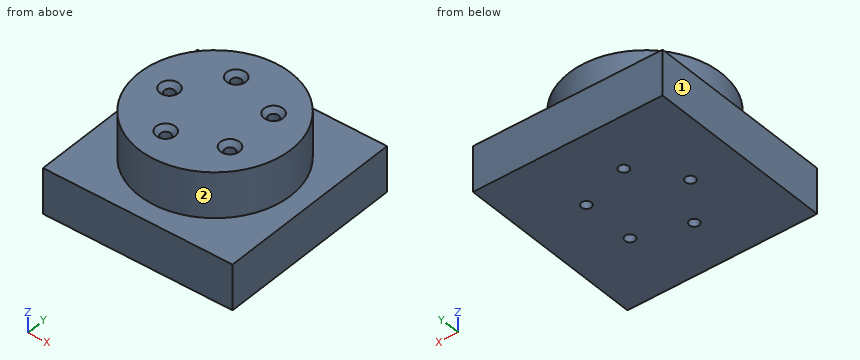
```python
from build123d import *

# Parameters (mm, degrees)
SKETCH1_W                                       = 125
SKETCH1_H                                       = 125
BOSS_EXTRUDE1_DEPTH                             = 30
SKETCH1_3_R                                     = 50
BOSS_EXTRUDE2_DEPTH                             = 30
CSK_FOR_M6_FLAT_HEAD_MACHINE_SCREW1_D           = 6.6
CSK_FOR_M6_FLAT_HEAD_MACHINE_SCREW1_CSINK_D     = 12.6
CSK_FOR_M6_FLAT_HEAD_MACHINE_SCREW1_CSINK_ANGLE = 90
CIRPATTERN1_COUNT                               = 5


with BuildPart() as part:
    # Sketch1 → Boss-Extrude1 (new body)
    with BuildSketch(Plane.XY):
        Rectangle(SKETCH1_W, SKETCH1_H)
    extrude(amount=-BOSS_EXTRUDE1_DEPTH)

    # Sketch1_3 → Boss-Extrude2 (add)
    with BuildSketch(Plane.XY):
        Circle(SKETCH1_3_R)
    extrude(amount=BOSS_EXTRUDE2_DEPTH)

    # CSK for M6 Flat Head Machine Screw1 (through all)
    with Locations(Plane.XY.offset(30)):
        with Locations((-30, 0)):
            csk_for_m6_flat_head_machine_screw1 = CounterSinkHole(CSK_FOR_M6_FLAT_HEAD_MACHINE_SCREW1_D / 2, CSK_FOR_M6_FLAT_HEAD_MACHINE_SCREW1_CSINK_D / 2, counter_sink_angle=CSK_FOR_M6_FLAT_HEAD_MACHINE_SCREW1_CSINK_ANGLE)

    # CirPattern1: CSK for M6 Flat Head Machine Screw1 ×5 about axis
    cirpattern1_axis = Axis((0, 0, 0), (0, 0, 1))
    for i in range(1, CIRPATTERN1_COUNT):
        add(csk_for_m6_flat_head_machine_screw1.rotate(cirpattern1_axis, i * 360 / CIRPATTERN1_COUNT), mode=Mode.SUBTRACT)


solid = part.part
```
The model under review builds one solid part; all positions refer to its coordinate system, in mm. Face numbers are marked on the shaded views. A direction names the side the tool comes from. Give positions to 0.01 mm unless a question says otherwise; leave off trailing zeros. Order: outer loops, then holes, each group sorted by start corner. A loop starts at its lowest first (then second) coordinate and runs counter-clockwise, first axis right, second up. Notation, with made-up numbers: (32.25, -20.75) - (39.25, -20.75) arc R29 ccw to (39.25, 7.25) - close; hole circle Ø8 at (55, 86). An arc over 180 degrees is marked (long way). Use CSV: the item, a comma, the result in double quotes. Start each with the question number.
Q1. We need section A-A, the plane x = -30. Write out the cut boundary in (y, z).
Q2. To check wall thickness, follow line 1 along Y through (x, z) = (-30, -5.5); line 2 along X through (y, z) = (17.5, -25); line 3 along Y through (x, z) = (-8, -16.5). State the ranges of each line that lie inside material, in increasing order. Write a range as [from, to].
Q3. We need section B-B, the plane y = 0. Write out the cut boundary in (x, z), and give its area (4 significant figures).
Q4. We need section D-D, the plane z = 23.5. Write out the cut boundary in (x, y).
Q5. We need section C-C, the plane x = 0. Write out the cut boundary in (y, z).
Q6. Tool access review of the marked faces 1 and 2: name each direction out of +Z, -Z, +X, -X, +Y, -Y from which nothing blocks a thin tool from reaching the whole face with its end or side.
Q7. Clearance check with flat-ended pins moving along their axes: pin 1 Ø3 at (y, z) = (-9.5, 15.5) entering from -X; pin 2 Ø10.5 at (x, y) = (-9.27, 28.53) entering from +Z; pin 3 Ø5 at (x, z) = (44, 20) entering from -Y. State where each tip first meets the part, or that it passes through.
Outcome:
1,outline,"(-62.5, -30) - (-3.3, -30) - (-3.3, 27) - (-6.3, 30) - (-40, 30) - (-40, 0) - (-62.5, 0) - close; (3.3, -30) - (62.5, -30) - (62.5, 0) - (40, 0) - (40, 30) - (6.3, 30) - (3.3, 27) - close"
2,line 1,"y = [-62.5, -3.3], [3.3, 62.5]"
2,line 2,"x = [-62.5, 20.97], [27.57, 62.5]"
2,line 3,"y = [-62.5, -31.58], [-25.49, 25.49], [31.58, 62.5]"
3,outline,"(-62.5, -30) - (-33.3, -30) - (-33.3, 27) - (-36.3, 30) - (-50, 30) - (-50, 0) - (-62.5, 0) - close; (-26.7, -30) - (62.5, -30) - (62.5, 0) - (50, 0) - (50, 30) - (-23.7, 30) - (-26.7, 27) - close"
3,area,"6,345 mm^2"
4,outline,"circle Ø100 at (0, 0); hole circle Ø6.6 at (-30, 0); hole circle Ø6.6 at (-9.27, -28.53); hole circle Ø6.6 at (-9.27, 28.53); hole circle Ø6.6 at (24.27, -17.63); hole circle Ø6.6 at (24.27, 17.63)"
5,outline,"(-62.5, -30) - (62.5, -30) - (62.5, 0) - (50, 0) - (50, 30) - (-50, 30) - (-50, 0) - (-62.5, 0) - close"
6,face 1,"+Z, -Z, -X, +Y, -Y"
6,face 2,"+Z"
7,pin 1,"stops at x = -49.36"
7,pin 2,"stops at z = 28.95"
7,pin 3,"stops at y = -27.89"
